from build123d import *

# Parameters (mm, degrees)
BOSS_EXTRUDE1_DEPTH = 8
SKETCH2_R           = 180
BOSS_EXTRUDE2_DEPTH = 1
CUT_EXTRUDE1_REACH  = 10
SKETCH3_R           = 2
CUT_EXTRUDE2_REACH  = 11
SKETCH5_W           = 16
SKETCH5_H           = 10


with BuildPart() as part:
    # Sketch1 → Boss-Extrude1 (new body)
    with BuildSketch(Plane.XY):
        Polygon((5, 230), (5, 180), (-5, 180), (-5, 230), (-7, 230), (-157.684812205, 167.584307141), (-159.099025767, 166.170093579), (-123.743686708, 130.814754519), (-130.81475452, 123.743686708), (-166.170093579, 159.099025767), (-167.584307141, 157.684812205), (-230, 7), (-230, 5), (-180, 5), (-180, -5), (-230, -5), (-230, -7), (-167.584307141, -157.684812205), (-166.170093579, -159.099025767), (-130.81475452, -123.743686708), (-123.743686708, -130.81475452), (-159.099025767, -166.170093579), (-157.684812205, -167.584307141), (-7, -230), (-5, -230), (-5, -180), (5, -180), (5, -230), (7, -230), (157.684812205, -167.584307141), (159.099025767, -166.170093579), (123.743686708, -130.814754519), (130.81475452, -123.743686708), (166.170093579, -159.099025767), (167.584307141, -157.684812205), (230, -7), (230, -5), (180, -5), (180, 5), (230, 5), (230, 7), (167.584307141, 157.684812205), (166.170093579, 159.099025767), (130.81475452, 123.743686708), (123.743686708, 130.81475452), (159.099025767, 166.170093579), (157.684812205, 167.584307141), (7, 230), align=None)
    extrude(amount=BOSS_EXTRUDE1_DEPTH)

    # Sketch2 → Boss-Extrude2 (add)
    with BuildSketch(Plane.XY.offset(8)):
        Circle(SKETCH2_R)
    extrude(amount=BOSS_EXTRUDE2_DEPTH)

    # Sketch3 → Cut-Extrude1 (cut, up to next)
    with BuildSketch(Plane.XY.offset(8), mode=Mode.PRIVATE) as cut_extrude1_sk1:
        with Locations((107.397750993, 174.354514299)):
            Circle(SKETCH3_R)
    cut_extrude1_tool1 = extrude(cut_extrude1_sk1.sketch, amount=-CUT_EXTRUDE1_REACH, mode=Mode.PRIVATE) & part.part
    add(cut_extrude1_tool1.solids().sort_by_distance((107.397751, 174.354514, 8))[0], mode=Mode.SUBTRACT)
    # Sketch3 → Cut-Extrude1 (cut, up to next)
    with BuildSketch(Plane.XY.offset(8), mode=Mode.PRIVATE) as cut_extrude1_sk2:
        with Locations((47.34558138, 199.228937402)):
            Circle(SKETCH3_R)
    cut_extrude1_tool2 = extrude(cut_extrude1_sk2.sketch, amount=-CUT_EXTRUDE1_REACH, mode=Mode.PRIVATE) & part.part
    add(cut_extrude1_tool2.solids().sort_by_distance((47.345581, 199.228937, 8))[0], mode=Mode.SUBTRACT)
    # Sketch3 → Cut-Extrude1 (cut, up to next)
    with BuildSketch(Plane.XY.offset(8), mode=Mode.PRIVATE) as cut_extrude1_sk3:
        with Locations((199.228937402, 47.34558138)):
            Circle(SKETCH3_R)
    cut_extrude1_tool3 = extrude(cut_extrude1_sk3.sketch, amount=-CUT_EXTRUDE1_REACH, mode=Mode.PRIVATE) & part.part
    add(cut_extrude1_tool3.solids().sort_by_distance((199.228937, 47.345581, 8))[0], mode=Mode.SUBTRACT)
    # Sketch3 → Cut-Extrude1 (cut, up to next)
    with BuildSketch(Plane.XY.offset(8), mode=Mode.PRIVATE) as cut_extrude1_sk4:
        with Locations((174.354514299, 107.397750993)):
            Circle(SKETCH3_R)
    cut_extrude1_tool4 = extrude(cut_extrude1_sk4.sketch, amount=-CUT_EXTRUDE1_REACH, mode=Mode.PRIVATE) & part.part
    add(cut_extrude1_tool4.solids().sort_by_distance((174.354514, 107.397751, 8))[0], mode=Mode.SUBTRACT)
    # Sketch3 → Cut-Extrude1 (cut, up to next)
    with BuildSketch(Plane.XY.offset(8), mode=Mode.PRIVATE) as cut_extrude1_sk5:
        with Locations((174.354514299, -107.397750993)):
            Circle(SKETCH3_R)
    cut_extrude1_tool5 = extrude(cut_extrude1_sk5.sketch, amount=-CUT_EXTRUDE1_REACH, mode=Mode.PRIVATE) & part.part
    add(cut_extrude1_tool5.solids().sort_by_distance((174.354514, -107.397751, 8))[0], mode=Mode.SUBTRACT)
    # Sketch3 → Cut-Extrude1 (cut, up to next)
    with BuildSketch(Plane.XY.offset(8), mode=Mode.PRIVATE) as cut_extrude1_sk6:
        with Locations((199.228937402, -47.34558138)):
            Circle(SKETCH3_R)
    cut_extrude1_tool6 = extrude(cut_extrude1_sk6.sketch, amount=-CUT_EXTRUDE1_REACH, mode=Mode.PRIVATE) & part.part
    add(cut_extrude1_tool6.solids().sort_by_distance((199.228937, -47.345581, 8))[0], mode=Mode.SUBTRACT)
    # Sketch3 → Cut-Extrude1 (cut, up to next)
    with BuildSketch(Plane.XY.offset(8), mode=Mode.PRIVATE) as cut_extrude1_sk7:
        with Locations((47.34558138, -199.228937402)):
            Circle(SKETCH3_R)
    cut_extrude1_tool7 = extrude(cut_extrude1_sk7.sketch, amount=-CUT_EXTRUDE1_REACH, mode=Mode.PRIVATE) & part.part
    add(cut_extrude1_tool7.solids().sort_by_distance((47.345581, -199.228937, 8))[0], mode=Mode.SUBTRACT)
    # Sketch3 → Cut-Extrude1 (cut, up to next)
    with BuildSketch(Plane.XY.offset(8), mode=Mode.PRIVATE) as cut_extrude1_sk8:
        with Locations((107.397750993, -174.354514299)):
            Circle(SKETCH3_R)
    cut_extrude1_tool8 = extrude(cut_extrude1_sk8.sketch, amount=-CUT_EXTRUDE1_REACH, mode=Mode.PRIVATE) & part.part
    add(cut_extrude1_tool8.solids().sort_by_distance((107.397751, -174.354514, 8))[0], mode=Mode.SUBTRACT)
    # Sketch3 → Cut-Extrude1 (cut, up to next)
    with BuildSketch(Plane.XY.offset(8), mode=Mode.PRIVATE) as cut_extrude1_sk9:
        with Locations((-107.397750993, -174.354514299)):
            Circle(SKETCH3_R)
    cut_extrude1_tool9 = extrude(cut_extrude1_sk9.sketch, amount=-CUT_EXTRUDE1_REACH, mode=Mode.PRIVATE) & part.part
    add(cut_extrude1_tool9.solids().sort_by_distance((-107.397751, -174.354514, 8))[0], mode=Mode.SUBTRACT)
    # Sketch3 → Cut-Extrude1 (cut, up to next)
    with BuildSketch(Plane.XY.offset(8), mode=Mode.PRIVATE) as cut_extrude1_sk10:
        with Locations((-47.34558138, -199.228937402)):
            Circle(SKETCH3_R)
    cut_extrude1_tool10 = extrude(cut_extrude1_sk10.sketch, amount=-CUT_EXTRUDE1_REACH, mode=Mode.PRIVATE) & part.part
    add(cut_extrude1_tool10.solids().sort_by_distance((-47.345581, -199.228937, 8))[0], mode=Mode.SUBTRACT)
    # Sketch3 → Cut-Extrude1 (cut, up to next)
    with BuildSketch(Plane.XY.offset(8), mode=Mode.PRIVATE) as cut_extrude1_sk11:
        with Locations((-199.228937402, -47.34558138)):
            Circle(SKETCH3_R)
    cut_extrude1_tool11 = extrude(cut_extrude1_sk11.sketch, amount=-CUT_EXTRUDE1_REACH, mode=Mode.PRIVATE) & part.part
    add(cut_extrude1_tool11.solids().sort_by_distance((-199.228937, -47.345581, 8))[0], mode=Mode.SUBTRACT)
    # Sketch3 → Cut-Extrude1 (cut, up to next)
    with BuildSketch(Plane.XY.offset(8), mode=Mode.PRIVATE) as cut_extrude1_sk12:
        with Locations((-174.354514299, -107.397750993)):
            Circle(SKETCH3_R)
    cut_extrude1_tool12 = extrude(cut_extrude1_sk12.sketch, amount=-CUT_EXTRUDE1_REACH, mode=Mode.PRIVATE) & part.part
    add(cut_extrude1_tool12.solids().sort_by_distance((-174.354514, -107.397751, 8))[0], mode=Mode.SUBTRACT)
    # Sketch3 → Cut-Extrude1 (cut, up to next)
    with BuildSketch(Plane.XY.offset(8), mode=Mode.PRIVATE) as cut_extrude1_sk13:
        with Locations((-174.354514299, 107.397750993)):
            Circle(SKETCH3_R)
    cut_extrude1_tool13 = extrude(cut_extrude1_sk13.sketch, amount=-CUT_EXTRUDE1_REACH, mode=Mode.PRIVATE) & part.part
    add(cut_extrude1_tool13.solids().sort_by_distance((-174.354514, 107.397751, 8))[0], mode=Mode.SUBTRACT)
    # Sketch3 → Cut-Extrude1 (cut, up to next)
    with BuildSketch(Plane.XY.offset(8), mode=Mode.PRIVATE) as cut_extrude1_sk14:
        with Locations((-199.228937402, 47.34558138)):
            Circle(SKETCH3_R)
    cut_extrude1_tool14 = extrude(cut_extrude1_sk14.sketch, amount=-CUT_EXTRUDE1_REACH, mode=Mode.PRIVATE) & part.part
    add(cut_extrude1_tool14.solids().sort_by_distance((-199.228937, 47.345581, 8))[0], mode=Mode.SUBTRACT)
    # Sketch3 → Cut-Extrude1 (cut, up to next)
    with BuildSketch(Plane.XY.offset(8), mode=Mode.PRIVATE) as cut_extrude1_sk15:
        with Locations((-47.34558138, 199.228937402)):
            Circle(SKETCH3_R)
    cut_extrude1_tool15 = extrude(cut_extrude1_sk15.sketch, amount=-CUT_EXTRUDE1_REACH, mode=Mode.PRIVATE) & part.part
    add(cut_extrude1_tool15.solids().sort_by_distance((-47.345581, 199.228937, 8))[0], mode=Mode.SUBTRACT)
    # Sketch3 → Cut-Extrude1 (cut, up to next)
    with BuildSketch(Plane.XY.offset(8), mode=Mode.PRIVATE) as cut_extrude1_sk16:
        with Locations((-107.397750993, 174.354514299)):
            Circle(SKETCH3_R)
    cut_extrude1_tool16 = extrude(cut_extrude1_sk16.sketch, amount=-CUT_EXTRUDE1_REACH, mode=Mode.PRIVATE) & part.part
    add(cut_extrude1_tool16.solids().sort_by_distance((-107.397751, 174.354514, 8))[0], mode=Mode.SUBTRACT)

    # Sketch5 → Cut-Extrude2 (cut, up to next)
    with BuildSketch(Plane(origin=(0, 0, 0), x_dir=(-1, 0, 0), z_dir=(0, 0, -1)), mode=Mode.PRIVATE) as cut_extrude2_sk1:
        with Locations((-24.221028692, -19.442057383)):
            Rectangle(SKETCH5_W, SKETCH5_H)
    cut_extrude2_tool1 = extrude(cut_extrude2_sk1.sketch, amount=-CUT_EXTRUDE2_REACH, mode=Mode.PRIVATE) & part.part
    add(cut_extrude2_tool1.solids().sort_by_distance((24.221029, -19.442057, 0))[0], mode=Mode.SUBTRACT)
    # Sketch5 → Cut-Extrude2 (cut, up to next)
    with BuildSketch(Plane(origin=(0, 0, 0), x_dir=(-1, 0, 0), z_dir=(0, 0, -1)), mode=Mode.PRIVATE) as cut_extrude2_sk2:
        with Locations((-24.221028692, 20.557942617)):
            Rectangle(SKETCH5_W, SKETCH5_H)
    cut_extrude2_tool2 = extrude(cut_extrude2_sk2.sketch, amount=-CUT_EXTRUDE2_REACH, mode=Mode.PRIVATE) & part.part
    add(cut_extrude2_tool2.solids().sort_by_distance((24.221029, 20.557943, 0))[0], mode=Mode.SUBTRACT)
    # Sketch5 → Cut-Extrude2 (cut, up to next)
    with BuildSketch(Plane(origin=(0, 0, 0), x_dir=(-1, 0, 0), z_dir=(0, 0, -1)), mode=Mode.PRIVATE) as cut_extrude2_sk3:
        with Locations((24.778971308, 20.557942617)):
            Rectangle(SKETCH5_W, SKETCH5_H)
    cut_extrude2_tool3 = extrude(cut_extrude2_sk3.sketch, amount=-CUT_EXTRUDE2_REACH, mode=Mode.PRIVATE) & part.part
    add(cut_extrude2_tool3.solids().sort_by_distance((-24.778971, 20.557943, 0))[0], mode=Mode.SUBTRACT)
    # Sketch5 → Cut-Extrude2 (cut, up to next)
    with BuildSketch(Plane(origin=(0, 0, 0), x_dir=(-1, 0, 0), z_dir=(0, 0, -1)), mode=Mode.PRIVATE) as cut_extrude2_sk4:
        with Locations((24.778971308, -19.442057383)):
            Rectangle(SKETCH5_W, SKETCH5_H)
    cut_extrude2_tool4 = extrude(cut_extrude2_sk4.sketch, amount=-CUT_EXTRUDE2_REACH, mode=Mode.PRIVATE) & part.part
    add(cut_extrude2_tool4.solids().sort_by_distance((-24.778971, -19.442057, 0))[0], mode=Mode.SUBTRACT)


solid = part.part
Input: part model. Units: mm. Frame: model coordinates. A direction names the side the tool comes from. Round coordinates to 2 decimals unless told otherwise and drop trailing zeros. Order: outer loops, then holes, each group sorted by start corner. A loop starts at its lowest first (then second) coordinate and runs counter-clockwise, first axis right, second up.
1. Mould query, pull axis X, two halves, no side actions, for faces 4 (the face through (-83.397, -198.355, 3.944)), 5 (the face through (141.67, -148.74, 3.94)), 6 (the face through (78, 179, 8)). Classes: released by +X, released by -X, zero draft, split by the parting line, or undercut.
The answers:
face 4: released by -X
face 5: undercut
face 6: zero draft
2. Material intervals for line 1 (Y direction, x = 150, z = 3); line 2 (X direction, y = -132.5, z = 7); line 3 (Y direction, x = -19, z = 1.75), sorted ascending.
The answers:
line 1: y = -170.77 to -157.07, -142.93 to 142.93, 157.07 to 170.77
line 2: x = -178.02 to -139.57, -125.43 to 125.43, 139.57 to 178.02
line 3: y = -225.03 to -24.44, -14.44 to 15.56, 25.56 to 225.03
3. Pin query (flat end, axial travel): P1, Ø2, axis at x = 72.5, z = 3.5, coming from the -Y side; P2, Ø12, axis at x = -112, y = 63, coming from the -Z side; P3, Ø4.5, axis at x = 107.4, y = 174.35, coming from the +Z side; P4, Ø2.5, axis at x = -27.5, z = 6.5, coming from the -Y side. Return the tip coordinate at first contact, or that it passes through.
The answers:
P1: stops at y = -203.28
P2: stops at z = 0
P3: stops at z = 8
P4: stops at y = -222.03
4. Cut plane A-A, the plane y = 62. Output: boundary loops of the cut face in (x, z).
The answers:
outline: (-207.22, 0) - (207.22, 0) - (207.22, 8) - (168.99, 8) - (168.99, 9) - (-168.99, 9) - (-168.99, 8) - (-207.22, 8) - close
5. Cut plane B-B, the plane x = 69. Output: boundary loops of the cut face in (y, z).
The answers:
outline: (-204.32, 0) - (204.32, 0) - (204.32, 8) - (166.25, 8) - (166.25, 9) - (-166.25, 9) - (-166.25, 8) - (-204.32, 8) - close
6. Cut plane C-C, the plane z = 3.25. State how many separate pieces and enclosed holes the cut face has, then the cut area to 3 significant figures.
The answers:
separate pieces: 1
enclosed holes: 20
area: 148,000 mm2
7. Set-up query: faces 1 (the face through (178, 81, 8)), 2 (the face through (178, -78, 8)), 3 (the face through (-179, 81, 8)). Return all of +Z, -Z, +X, -X, +Y, -Y with unobstructed straight access to the full face (end or side cutting, diameter ignored); none if empty.
The answers:
face 1: +Z, +X, +Y
face 2: +Z, +X, -Y
face 3: +Z, -X, +Y
